Could you check a few things on this model? Use its own coordinates, in mm. A direction names the side the tool comes from. Give positions to 0.01 mm unless a question says otherwise; leave off trailing zeros. Answer as a JSON object with one key per item and string values. Group by question number.
Autodesk Inventor part; units mm, degrees
ref_plane "YZ Plane" through (0, 0, 0) normal (1, 0, 0) x (0, 1, 0)
ref_plane "XZ Plane" through (0, 0, 0) normal (0, 1, 0) x (-1, 0, 0)
ref_plane "XY Plane" through (0, 0, 0) normal (0, 0, 1) x (1, 0, 0)
sketch "Náčrt1" plane through (0, 0, 0) normal (0, 0, 1) x (1, 0, 0)
  circle A0 centre (0, 0) radius 2.5
  line L0 (-1.5, -2.5) -> (1.5, -2.5)
  line L1 (1.5, -2.5) -> (1.5, 2.5)
  line L2 (1.5, 2.5) -> (-1.5, 2.5)
  line L3 (-1.5, 2.5) -> (-1.5, -2.5)
  line L4 (-1.5, -2.5) -> (1.5, 2.5) construction
  line L5 (1.5, -2.5) -> (-1.5, 2.5) construction
  circle A1 centre (0, 0) radius 15
  point P0 (-1.5, -2)
  point P1 (-1.5, 2)
  point P2 (1.5, 2)
  point P3 (1.5, -2)
  dimension "d0" = 5
  dimension "d1" = 3
  dimension "d2" = 5
  dimension "d3" = 30
extrude "Vysunutí1" add sketch "Náčrt1" along normal mid plane 6 contours A0 L1 | A0 L2 L1 | L1 L0 A0 | A0 L3 L2 | L0 L3 A0 | L3 A0 | A1
sketch "Náčrt2" plane through (0, 0, 0) normal (1, 0, 0) x (0, 1, 0)
  line L0 (-15, -3) -> (15, -3)
  line L1 (15, 3) -> (15, -3)
  line L2 (15, -3) -> (13.2124, -1.5)
  line L3 (15, -3) -> (17.3336, -3) construction
  line L4 (15, 3) -> (-15, 3)
  line L5 (15, 3) -> (13.2124, 1.5)
  line L6 (15, 3) -> (17.3336, 3) construction
  line L7 (13.2124, 1.5) -> (13.2124, -1.5)
  line L8 (0, -7) -> (0, 7)
  point P0 (0, 0)
  dimension "d15" = 140
  dimension "d16" = 140
  dimension "d18" = 3
  dimension "d27" = 13.2124
  dimension "d28" = 1.5
revolve "Rotace1" cut sketch "Náčrt2" angle 360 about axis through (0, 0, -10) along (0, 0, 1) contours L2 L7 L5 L1
fillet "Zaoblení1" radius 0.5 2 edges at (0, -15, -3) (0, -15, 3)
sketch "Náčrt3" plane through (0, 0, 3) normal (0, 0, 1) x (1, 0, 0)
  circle A0 centre (0, 0) radius 3.5
  circle A1 centre (0, 0) radius 10
  dimension "d12" = 7
  dimension "d13" = 20
extrude "Vysunutí2" cut sketch "Náčrt3" against normal blind 3
chamfer "Zkosení1" distance 3 angle 45 1 edges at (-10, 0, 3)
chamfer "Zkosení2" distance 3 angle 45 1 edges at (-3.5, 0, 0)
equation "\"d15\" = d16"
properties part number "rub-ring_3D tisk"
(1) Will these pins go through, and if not, where does the flat tip stop? P1, Ø1.5, axis at x = 8.5, z = 1, coming from the +Y side; P2, Ø16, axis at x = 0, y = 0, coming from the -Z side; P3, Ø5, axis at x = 6.5, y = 5, coming from the +Z side; P4, Ø3, axis at y = 0.5, z = 1, coming from the +X side.
(2) For faces 4 (the flat face through (0, -3, -3)), 5 (the flat face through (1.5, 0, 0)), which set-ups out of +Z, -Z, +X, -X, +Y, -Y let a thin tool reach every point of the face, with its end or its side?
(3) If we mould it in two halves opening along Z, with no side actions, what happens to faces 1 (the flat face through (7, 0, 0)), 2 (the flat face through (-1.5, 0, 0)), 3 (the cylindrical face through (-8.04, -10.485, -0.021))? For each: +Z half, -Z half, draft (parallel to the pull), parting line (faces both ways), or undercut.
(4) I need wall thicknesses on L1, parallel to Y at x = 0, z = 0.05; L2, parallel to Y at x = 0, z = -0.3; L3, parallel to Z at x = -9.75, y = 10. Which ranges of each line are inside material? Lowest first, please.
Entries:
{
 "1": {"P1": "y = 10.7", "P2": "z = -3", "P3": "z = 0.8", "P4": "x = 14.12"},
 "2": {"face 4": "-Z, +X, -X, +Y, -Y", "face 5": "+Z, -Z"},
 "3": {"face 1": "+Z half", "face 2": "draft", "face 3": "undercut"},
 "4": {"L1": "-13.21 to -10.05, -6.45 to -2.5, 2.5 to 6.45, 10.05 to 13.21", "L2": "-13.21 to -2.5, 2.5 to 13.21", "L3": "-2.87 to -2.13, 2.13 to 2.87"}
}
